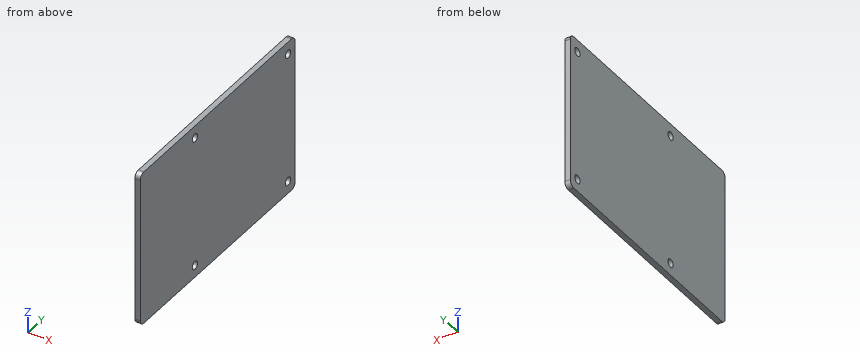
from build123d import *

# Parameters (mm, degrees)
F0_W     = 88
F0_H     = 57
F0_R     = 1.5
F1_DEPTH = 2
F2_R     = 2


with BuildPart() as f1:
    # F0 (on Right) → F1 (new body)
    with BuildSketch(Plane.YZ):
        with Locations((44, 28.5)):
            Rectangle(F0_W, F0_H)
        with Locations((31, 4.5)):
            Circle(F0_R, mode=Mode.SUBTRACT)
        with Locations((84, 4.5)):
            Circle(F0_R, mode=Mode.SUBTRACT)
        with Locations((31, 52.5)):
            Circle(F0_R, mode=Mode.SUBTRACT)
        with Locations((84, 52.5)):
            Circle(F0_R, mode=Mode.SUBTRACT)
    extrude(amount=F1_DEPTH)

    # F2
    f2_edges = [f1.edges().sort_by_distance(p)[0] for p in [
        (1, 0, 0),
        (1, 88, 0),
        (1, 0, 57),
        (1, 88, 57),
    ]]
    fillet(f2_edges, radius=F2_R)


solid = f1.part
Model file for the job. Use its own axes, mm. Give positions to 0.01 mm unless a question says otherwise; leave off trailing zeros. Order: outer loops, then holes, each group sorted by start corner. A loop starts at its lowest first (then second) coordinate and runs counter-clockwise, first axis right, second up. Notation, with made-up numbers: (-25.75, 17) - (5.25, 17) arc R21 cw to (5.25, 45) - close; hole circle Ø2 at (-38, 70.25). An arc over 180 degrees is marked (long way). Return JSON: item names as keys, results as strings.
1) Probe line 1 (Z direction, x = 1, y = 31); line 2 (Y direction, x = 0.3, z = 5); line 3 (Y direction, x = 1.6, z = 53.5). List the from-to ranges inside material, lowest first. Write a range as from..to.
Geometry says:
{"line 1": "0..3, 6..51, 54..57", "line 2": "0..29.59, 32.41..82.59, 85.41..88", "line 3": "0..29.88, 32.12..82.88, 85.12..88"}
2) Flat gauge pin, fed straight in: P1, Ø2.5, axis at y = 31, z = 52.5, coming from the -X side. Where does the tip first touch, or does it go through?
Geometry says:
{"P1": "through"}
3) Cut at A-A, the plane y = 84. Give the cut face in (x, z).
Geometry says:
{"outline": "(0, 0) - (2, 0) - (2, 3) - (0, 3) - close; (0, 6) - (2, 6) - (2, 51) - (0, 51) - close; (0, 54) - (2, 54) - (2, 57) - (0, 57) - close"}
